Design review of the part shown in the three views and the two pictorial views. Dimensions are in mm from the part's minimum x, y and z. A direction names the side the tool comes from. Round coordinates to 2 decimals unless told otherwise and drop trailing zeros. Loops run counter-clockwise (first coordinate to the right, second up) from the corner with the lowest first, then second, coordinate; pieces in that order, holes last. Notation, with made-up numbers: (-21, 54) -> (11, 54) arc R15 ccw to (11, 65) -> close; hole circle Ø11 at (16, 27.5). An arc over 180 degrees is marked (long way). One line per question, with ' | ' between items. Start each with the question number.
1. For the marked faces 4, 5 and 6, list the 3-axis set-ups (+Z, -Z, +X, -X, +Y, -Y) from which the entire face can be reached by the end or side of a thin tool; tool diameter is ignored.
2. Consider section C-C (x = 2). Write out the cut boundary in (y, z).
3. Draft analysis for pull direction Z (two halves, no side actions). For the marked faces 1, 2 and 3, state which applies: pulls with the +Z half, pulls with the -Z half, needs draft (parallel to the pull), parting line crosses it, or undercut.
4. For pin 1 Ø0.6 at (x, z) = (16, 3.5) entering from -Y; pin 2 Ø3 at (x, y) = (7.5, 6) entering from +Z; pin 3 Ø0.7 at (x, z) = (15.9, 3.9) entering from -Y, all flat-tipped, find the tip position at first contact; note any pin that passes through.
5. Consider section D-D (x = 15.9). Write out the cut boundary in (y, z), and give its area (3 significant figures).
6. Consider section B-B (z = 3.9). Write out the cut boundary in (x, y).
7. Consider section A-A (y = 1.25). Write out the cut boundary in (x, z).
8. Wall thickness on line 1 along X through (y, z) = (0.8, 3.9); line 2 along Z through (x, y) = (8, 1.5); line 3 along Y through (x, z) = (1, 7.25): over which ranges is each line inside the solid? List them lowest first.
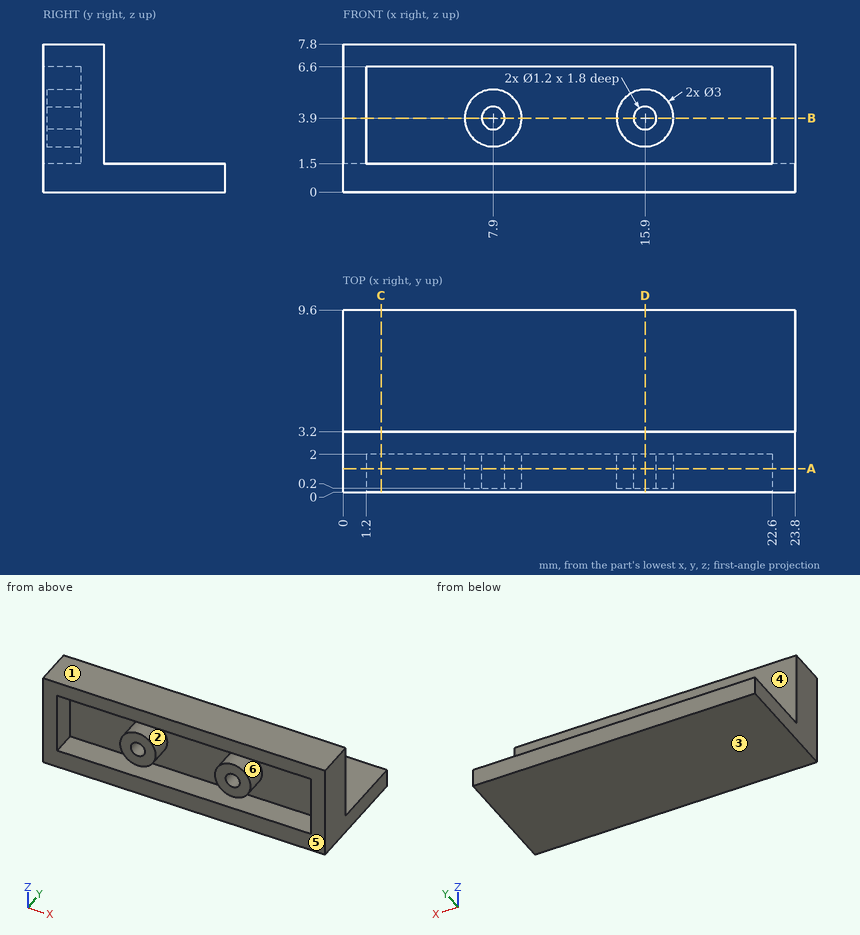
Answer block:
1) face 4: +Z, +X, -X, +Y | face 5: +Z, -Z, +X, -X, -Y | face 6: -Y
2) outline: (0, 0) -> (9.6, 0) -> (9.6, 1.5) -> (3.2, 1.5) -> (3.2, 7.8) -> (0, 7.8) -> (0, 6.6) -> (2, 6.6) -> (2, 1.5) -> (0, 1.5) -> close
3) face 1: pulls with the +Z half | face 2: undercut | face 3: pulls with the -Z half
4) pin 1: stops at y = 0.2 | pin 2: stops at z = 1.5 | pin 3: stops at y = 2
5) outline: (0, 0) -> (9.6, 0) -> (9.6, 1.5) -> (3.2, 1.5) -> (3.2, 7.8) -> (0, 7.8) -> (0, 6.6) -> (2, 6.6) -> (2, 5.4) -> (0.2, 5.4) -> (0.2, 4.5) -> (2, 4.5) -> (2, 3.3) -> (0.2, 3.3) -> (0.2, 2.4) -> (2, 2.4) -> (2, 1.5) -> (0, 1.5) -> close | area: 27.6 mm2
6) outline: (0, 0) -> (1.2, 0) -> (1.2, 2) -> (6.4, 2) -> (6.4, 0.2) -> (7.3, 0.2) -> (7.3, 2) -> (8.5, 2) -> (8.5, 0.2) -> (9.4, 0.2) -> (9.4, 2) -> (14.4, 2) -> (14.4, 0.2) -> (15.3, 0.2) -> (15.3, 2) -> (16.5, 2) -> (16.5, 0.2) -> (17.4, 0.2) -> (17.4, 2) -> (22.6, 2) -> (22.6, 0) -> (23.8, 0) -> (23.8, 3.2) -> (0, 3.2) -> close
7) outline: (0, 0) -> (23.8, 0) -> (23.8, 7.8) -> (0, 7.8) -> close; circle Ø3 at (7.9, 3.9); circle Ø3 at (15.9, 3.9); hole (1.2, 1.5) -> (22.6, 1.5) -> (22.6, 6.6) -> (1.2, 6.6) -> close; hole circle Ø1.2 at (7.9, 3.9); hole circle Ø1.2 at (15.9, 3.9)
8) line 1: x = 0 to 1.2, 6.4 to 7.3, 8.5 to 9.4, 14.4 to 15.3, 16.5 to 17.4, 22.6 to 23.8 | line 2: z = 0 to 1.5, 2.4 to 3.31, 4.49 to 5.4, 6.6 to 7.8 | line 3: y = 0 to 3.2
